```python
from build123d import *

# Parameters (mm, degrees)
F1_DEPTH = 71.4375
F2_R     = 1.9812
F3_DEPTH = 6.096
F5_DEPTH = 31.243


# Not quite as in the source:
# - a feature names something its author has since deleted; it is built from what else it names


with BuildPart() as f1:
    # F0 (on Front) → F1 (new body)
    with BuildSketch(Plane.XZ):
        Polygon((3.1813341729, 6.0924417882), (3.1813341729, 12.1884417882), (-2.9146658271, 12.1884417882), (-2.9146658271, -1.2735582118), (28.3273341729, -1.2735582118), (28.3273341729, 12.1884417882), (22.2313341729, 12.1884417882), (22.2313341729, 6.0924417882), (24.3903341729, 6.0924417882), (24.3903341729, 2.5364417882), (1.0223341729, 2.5364417882), (1.0223341729, 6.0924417882), align=None)
    extrude(amount=F1_DEPTH)

    # F2 (on face) → F3 (cut, through all)
    with BuildSketch(Plane.YZ.offset(28.3273341729)):
        with Locations((-58.1025, 8.7594417882)):
            Circle(F2_R)
    extrude(amount=-F3_DEPTH, mode=Mode.SUBTRACT)

    # F4 (on face) → F5 (cut, through all)
    with BuildSketch(Plane.YZ.offset(28.3273341729)):
        with BuildLine():
            ThreePointArc((0, -1.2735582118), (-35.71875, 1.0124417882), (-71.4375, -1.2735582118))
            Line((-71.4375, -1.2735582118), (0, -1.2735582118))
        make_face()
    extrude(amount=-F5_DEPTH, mode=Mode.SUBTRACT)


solid = f1.part
```
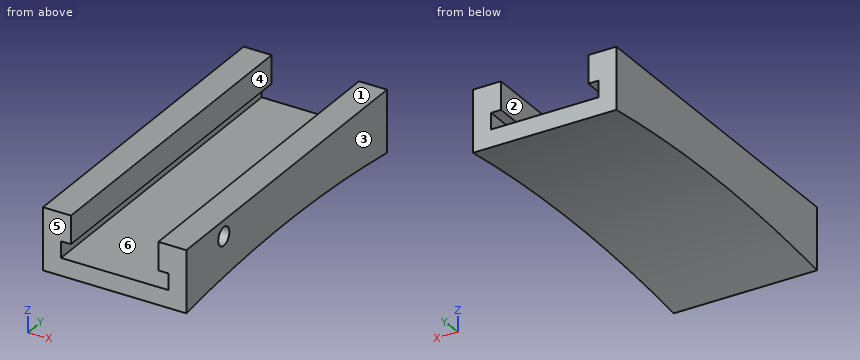
Source: CAD feature listing. Evaluate the final solid. Frame: model axes, mm. Face numbers are marked on the shaded views. A direction names the side the tool comes from. Round coordinates to 2 decimals unless told otherwise and drop trailing zeros. Loops run counter-clockwise (first coordinate to the right, second up) from the corner with the lowest first, then second, coordinate; pieces in that order, holes last. Notation, with made-up numbers: M 64,0 L 113,0 A17 ccw 113,22 Z; hole C 82.25,-1 d5. An arc over 180 degrees is marked long. Use a Markdown table: item, result. Add a question column.
1. Section query D-D on x = 19. Return the cut outline in (y, z), then the cut area to 3 significant figures.
2. Mould query, pull axis X, two halves, no side actions, for the marked faces 3, 4, 5 and 6. Classes: pulls with the +X half, pulls with the -X half, needs draft (parallel to the pull), parting line crosses it, or undercut.
3. Section query A-A on y = -59. Return the cut outline in (x, z).
4. Line query: line 1 (X direction, y = -5.5, z = 10.75); line 2 (X direction, y = -43, z = 5.75); line 3 (Z direction, x = 2, y = -57). Output: solid intervals per line, ascending.
5. Reachability of the marked faces 1 and 2 from +Z, -Z, +X, -X, +Y, -Y: full face, straight path, thin tool, end or side. Return the list, or none.
6. Contact query for flat-ended pins moving along their axis: P1, Ø3, axis at x = 20.5, y = -64, coming from the +Z side; P2, Ø1.5, axis at x = 4, y = -51.5, coming from the -Z side; P3, Ø0.6, axis at x = 1.5, y = -25.5, coming from the -Z side; P4, Ø2, axis at x = 24, z = 3.5, coming from the +Y side. Output: stop coordinate, or through.
7. Section query C-C on y = -25. Return the cut outline in (x, z), then the cut area to 3 significant figures.
Reported:
| question | item | result |
|---|---|---|
| 1 | outline | M -71.44,-1.27 A280.2 cw 0,-1.27 L 0,2.54 L -71.44,2.54 Z |
| 1 | area | 163 mm² |
| 2 | face 3 | pulls with the +X half |
| 2 | face 4 | undercut |
| 2 | face 5 | needs draft |
| 2 | face 6 | undercut |
| 3 | outline | M -2.91,0.04 L 28.33,0.04 L 28.33,6.99 L 22.23,6.99 L 22.23,6.09 L 24.39,6.09 L 24.39,2.54 L 1.02,2.54 L 1.02,6.09 L 3.18,6.09 L 3.18,12.19 L -2.91,12.19 Z; M 22.23,10.53 L 28.33,10.53 L 28.33,12.19 L 22.23,12.19 Z |
| 4 | line 1 | x = -2.91 to 3.18, 22.23 to 28.33 |
| 4 | line 2 | x = -2.91 to 1.02, 24.39 to 28.33 |
| 4 | line 3 | z = 0.2 to 2.54, 6.09 to 12.19 |
| 5 | face 1 | +Z, +X, -X, +Y, -Y |
| 5 | face 2 | +Z, +Y, -Y |
| 6 | P1 | stops at z = 2.54 |
| 6 | P2 | stops at z = 0.52 |
| 6 | P3 | stops at z = 0.81 |
| 6 | P4 | stops at y = 0 |
| 7 | outline | M -2.91,0.81 L 28.33,0.81 L 28.33,12.19 L 22.23,12.19 L 22.23,6.09 L 24.39,6.09 L 24.39,2.54 L 1.02,2.54 L 1.02,6.09 L 3.18,6.09 L 3.18,12.19 L -2.91,12.19 Z |
| 7 | area | 156 mm² |
